Autodesk Inventor part; units mm, degrees
ref_plane "YZ Plane" through (0, 0, 0) normal (1, 0, 0) x (0, 1, 0)
ref_plane "XZ Plane" through (0, 0, 0) normal (0, 1, 0) x (-1, 0, 0)
ref_plane "XY Plane" through (0, 0, 0) normal (0, 0, 1) x (1, 0, 0)
sketch "Sketch1" plane through (0, 0, 0) normal (0, 1, 0) x (-1, 0, 0)
  line L0 (-5, 5) -> (5, 5)
  line L1 (5, 5) -> (5, -5)
  line L2 (5, -5) -> (-5, -5)
  line L3 (-5, -5) -> (-5, 5)
  line L4 (-5, 5) -> (5, -5) construction
  line L5 (5, 5) -> (-5, -5) construction
  point P0 (0, 0)
  dimension "d0" = 10
  dimension "d1" = 10
extrude "Extrusion1" add sketch "Sketch1" along normal blind 10
sketch "Sketch2" plane through (5, 0, 5) normal (1, 0, 0) x (0, 0, -1)
  line L0 (10, 10) -> (7.5, 10)
  line L1 (7.5, 10) -> (7.5, 2.5)
  line L2 (7.5, 2.5) -> (10, 2.5)
  line L3 (10, 2.5) -> (10, 10)
  point P0 (5, 0)
  dimension "d4" = 2.5
  dimension "d5" = 7.5
extrude "Extrusion2" cut sketch "Sketch2" against normal blind 10
sketch "Sketch3" plane through (5, 0, 5) normal (1, 0, 0) x (0, 0, -1)
  line L0 (7.5, 10) -> (5, 10)
  line L1 (5, 10) -> (5, 5)
  line L2 (5, 5) -> (7.5, 5)
  line L3 (7.5, 5) -> (7.5, 10)
  point P0 (5, 0)
  dimension "d8" = 2.5
  dimension "d9" = 5
extrude "Extrusion3" cut sketch "Sketch3" against normal blind 10
sketch "Sketch4" plane through (5, 0, 5) normal (1, 0, 0) x (0, 0, -1)
  line L0 (5, 10) -> (2.5, 10)
  line L1 (2.5, 10) -> (2.5, 7.5)
  line L2 (2.5, 7.5) -> (5, 7.5)
  line L3 (5, 7.5) -> (5, 10)
  point P0 (5, 0)
  dimension "d12" = 2.5
  dimension "d13" = 2.5
extrude "Extrusion4" cut sketch "Sketch4" against normal blind 10
sketch "Sketch5" plane through (-5, 0, 5) normal (0, 0, 1) x (1, 0, 0)
  line L0 (0, 10) -> (10, 10)
  line L1 (0, 0) -> (0, 10)
  line L2 (0, 10) -> (0, 2.5)
  line L3 (0, 2.5) -> (2.5, 2.5)
  line L4 (2.5, 2.5) -> (2.5, 5)
  line L5 (2.5, 5) -> (5, 5)
  line L6 (5, 5) -> (5, 7.5)
  line L7 (5, 7.5) -> (7.5, 7.5)
  line L8 (7.5, 7.5) -> (7.5, 10)
  point P0 (5, 0)
  dimension "d16" = 7.5
  dimension "d17" = 2.5
  dimension "d18" = 2.5
  dimension "d19" = 90
  dimension "d20" = 2.5
  dimension "d21" = 90
  dimension "d22" = 2.5
  dimension "d23" = 90
  dimension "d24" = 2.5
  dimension "d25" = 90
extrude "Extrusion5" cut sketch "Sketch5" against normal blind 10
properties part number "157"
Can you work these out from the model? Positions are in its coordinate system, mm. A direction names the side the tool comes from. Round coordinates to 2 decimals unless told otherwise and drop trailing zeros. Loops run counter-clockwise (first coordinate to the right, second up) from the corner with the lowest first, then second, coordinate; pieces in that order, holes last.
Item 1: Please list where these lines run through material, in increasing order: L1, parallel to Y at x = 4, z = -2.25; L2, parallel to Z at x = 3.75, y = 3.5; L3, parallel to Y at x = 1.75, z = -3.5.
Item 2: Suppose I cut it at B-B, the plane z = 1.75. Write out the boundary of the cut face in (x, y).
Item 3: Suppose I cut it at A-A, the plane x = 4. Write out the boundary of the cut face in (y, z).
Item 4: Will these pins go through, and if not, where does the flat tip stop? pin 1 Ø1.2 at (x, y) = (3.5, 9.5) entering from -Z; pin 2 Ø1.2 at (y, z) = (3.5, 0.5) entering from -X; pin 3 Ø1.2 at (x, y) = (3, 6.5) entering from -Z.
Item 5: Which directions (+Z, -Z, +X, -X, +Y, -Y) give clear straight access to the entire face, cutting with the end or side of a thin tool? Please do faces 1 (the flat face through (1, 4, 5)), 2 (the flat face through (1, 4, -2.5)), 3 (the flat face through (-2.5, 4, 1)).
Item 6: Suppose I cut it at C-C, the plane y = 8.75. Write out the boundary of the cut face in (x, z), then the cut area to 3 significant figures.
Item 7: Suppose I cut it at D-D, the plane x = 1. Write out the boundary of the cut face in (y, z), then the cut area to 4 significant figures.
Reported:
1. L1: y = 0 to 5
1. L2: z = -2.5 to 5
1. L3: y = 0 to 2.5
2. outline: (-5, 0) - (5, 0) - (5, 7.5) - (0, 7.5) - (0, 5) - (-2.5, 5) - (-2.5, 2.5) - (-5, 2.5) - close
3. outline: (0, -5) - (2.5, -5) - (2.5, -2.5) - (5, -2.5) - (5, 0) - (7.5, 0) - (7.5, 2.5) - (10, 2.5) - (10, 5) - (0, 5) - close
4. pin 1: stops at z = 2.5
4. pin 2: stops at x = -2.5
4. pin 3: stops at z = 0
5. face 1: +Z, +X, -X, +Y, -Y
5. face 2: -Z, +X, -X, +Y
5. face 3: +Z, -Z, -X, +Y
6. outline: (2.5, 2.5) - (5, 2.5) - (5, 5) - (2.5, 5) - close
6. area: 6.25 mm2
7. outline: (0, -5) - (2.5, -5) - (2.5, -2.5) - (5, -2.5) - (5, 0) - (7.5, 0) - (7.5, 5) - (0, 5) - close
7. area: 56.25 mm2
